The model under review builds one solid part; all positions refer to its coordinate system, in mm. A direction names the side the tool comes from. Coordinates: 2 decimals unless noted, no trailing zeros. Write each loop counter-clockwise with the first axis right and the second up, starting at its lowest first coordinate (ties: lowest second). Pieces come first, ordered by that corner, then holes. Notation, with made-up numbers: (-33, 11) - (-2, 11) arc R36 cw to (-2, 48) - close; hole circle Ø11 at (31, 74). An arc over 180 degrees is marked (long way). Put each result on its own line as item: value. Start each with the question number.
Item 1: To check wall thickness, follow L1, parallel to X at y = -12.5, z = 3.5; L2, parallel to Z at x = 15.4, y = -16; L3, parallel to Z at x = -2.5, y = -10. State the ranges of each line that lie inside material, in increasing order. Write a range as [from, to].
Item 2: Consider section D-D on y = -6.5. Give the boundary of the cut face in (x, z), then the cut area to 3 significant figures.
Item 3: Mouldability with a two-part tool opening along Z and no side actions: class faces 3 (the face through (16, -12, 0)), 4 (the face through (15.507, -13.577, 0.513)), 5 (the face through (-15.493, -13.577, 0.513)), 6 (the face through (0, -12, -16.25)) as pulls with the +Z half, pulls with the -Z half, needs draft (parallel to the pull), parting line crosses it, or undercut.
Item 4: Machinability: for faces 1 (the face through (-16, -12, 0)), 2 (the face through (4, -16, -15.25)), which of the approach directions +Z, -Z, +X, -X, +Y, -Y give a long, thin tool a straight path to every point of the face, cutting with its end or side? Answer none if there is none.
Item 5: Consider section A-A on z = 4.5. Give the boundary of the cut face in (x, y).
Item 6: Consider section B-B on y = -15. Give the boundary of the cut face in (x, z), then the cut area to 3 significant figures.
Item 7: For pin 1 (1.5 mm diameter, centred on x = 12.5, y = -15, fed in from +Z); pin 2 (6 mm diameter, centred on y = -16, z = -0.25, fed in from +X), all flat-tipped, find the tip position at first contact; note any pin that passes through.
Item 8: Consider section C-C on z = -0.25. Give the boundary of the cut face in (x, y), then the cut area to 3 significant figures.
```python
from build123d import *

# Parameters (mm, degrees)
F1_DEPTH = 32
F2_R     = 2.54
F3_DEPTH = 228.6
F5_DEPTH = 76.2


with BuildPart() as f1:
    # F0 (on Front) → F1 (new body)
    with BuildSketch(Plane.XZ):
        Polygon((-15, 15.75), (-16, 15.75), (-16, -16.25), (16, -16.25), (16, 15.75), (15, 15.75), (15, -15.25), (-15, -15.25), align=None)
    extrude(amount=F1_DEPTH)

    # F2 (on face) → F3 (cut)
    with BuildSketch(Plane.YZ.offset(16)):
        with Locations((-16, -0.25)):
            Circle(F2_R)
    extrude(amount=-F3_DEPTH, mode=Mode.SUBTRACT)

    # F4 (on face) → F5 (cut)
    with BuildSketch(Plane(origin=(0, 0, -16.25), x_dir=(1, 0, 0), z_dir=(0, 0, -1))):
        with BuildLine():
            Line((1.7960512242, 14.2039487758), (-1.7960512242, 17.7960512242))
            ThreePointArc((-1.7960512242, 17.7960512242), (-1.7960512242, 14.2039487758), (1.7960512242, 14.2039487758))
        make_face()
        with BuildLine():
            ThreePointArc((2.54, 16), (0.9720159182, 18.3466540126), (-1.7960512242, 17.7960512242))
            Line((-1.7960512242, 17.7960512242), (1.7960512242, 14.2039487758))
            ThreePointArc((1.7960512242, 14.2039487758), (2.3466540126, 15.0279840818), (2.54, 16))
        make_face()
    extrude(amount=-F5_DEPTH, mode=Mode.SUBTRACT)


solid = f1.part
```
Report:
1. L1: [-16, -15], [15, 16]
1. L2: [-16.25, -2.79], [2.29, 15.75]
1. L3: [-16.25, -15.25]
2. outline: (-16, -16.25) - (16, -16.25) - (16, 15.75) - (15, 15.75) - (15, -15.25) - (-15, -15.25) - (-15, 15.75) - (-16, 15.75) - close
2. area: 94.0 mm²
3. face 3: needs draft
3. face 4: undercut
3. face 5: undercut
3. face 6: pulls with the -Z half
4. face 1: +Z, -Z, -X, +Y, -Y
4. face 2: +Z, +Y, -Y
5. outline: (-16, -32) - (-15, -32) - (-15, 0) - (-16, 0) - close; (15, -32) - (16, -32) - (16, 0) - (15, 0) - close
6. outline: (-16, -16.25) - (-2.33, -16.25) - (-2.33, -15.25) - (-15, -15.25) - (-15, -2.58) - (-16, -2.58) - close; (-16, 2.08) - (-15, 2.08) - (-15, 15.75) - (-16, 15.75) - close; (2.33, -16.25) - (16, -16.25) - (16, -2.58) - (15, -2.58) - (15, -15.25) - (2.33, -15.25) - close; (15, 2.08) - (16, 2.08) - (16, 15.75) - (15, 15.75) - close
6. area: 80.0 mm²
7. pin 1: z = -15.25
7. pin 2: x = 16
8. outline: (-16, -32) - (-15, -32) - (-15, -18.54) - (-16, -18.54) - close; (-16, -13.46) - (-15, -13.46) - (-15, 0) - (-16, 0) - close; (15, -32) - (16, -32) - (16, -18.54) - (15, -18.54) - close; (15, -13.46) - (16, -13.46) - (16, 0) - (15, 0) - close
8. area: 53.8 mm²
